Input: part model. Units: mm. Frame: model coordinates. Coordinates: 2 decimals unless noted, no trailing zeros. Loops run counter-clockwise (first coordinate to the right, second up) from the corner with the lowest first, then second, coordinate; pieces in that order, holes last. Notation, with made-up numbers: (77, 38.5) -> (125, 38.5) arc R24 cw to (125, 64.5) -> close; hole circle Ø7 at (43.25, 39.5). An arc over 180 degrees is marked (long way). Put each result on its own line as item: value. Start each with the question number.
1) Cut plane B-B (y = -111.5). Return the cut outline in (x, z), plus the area to 3 significant figures.
2) Cut plane A-A (z = 2.35). Return the cut outline in (x, y), plus the area to 3 significant figures.
3) Material intervals for L1, parallel to X at y = -190, z = 0.4; L2, parallel to Y at x = 71.5, z = 1.25; L3, parallel to X at y = -83, z = 2.1, sorted ascending.
4) Cut plane C-C (x = 137). Return the cut outline in (y, z), plus the area to 3 significant figures.
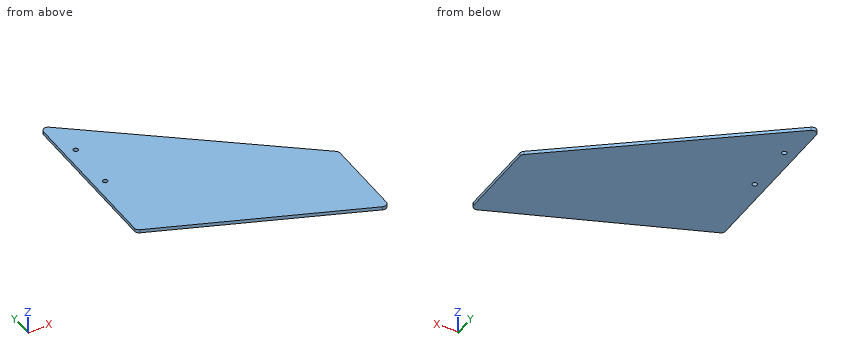
from build123d import *

# Parameters (mm, degrees)
EXTRUDE_1_DEPTH     = 3
FILLET_1_R          = 4
SKETCH_2_R          = 2.1
CUT_EXTRUDE_1_DEPTH = 3


with BuildPart() as part:
    # Эскиз1 → Бобышка-Вытянуть1 (new body)
    with BuildSketch(Plane.XY):
        Polygon((0, 0), (-3.068659699, -150), (178.455758645, -224), (180.065729767, -145.302558134), align=None)
    extrude(amount=EXTRUDE_1_DEPTH)

    # Скругление1
    fillet_1_edges = [part.edges().sort_by_distance(p)[0] for p in [
        (178.455758645, -224, 1.5),
        (-3.068659699, -150, 1.5),
        (0, 0, 1.5),
        (180.065729767, -145.302558134, 1.5),
    ]]
    fillet(fillet_1_edges, radius=FILLET_1_R)

    # Эскиз2 → Вырез-Вытянуть1 (cut)
    with BuildSketch(Plane.XY.offset(3)):
        with Locations((9.183783122, -40)):
            Circle(SKETCH_2_R)
        with Locations((8.259287105, -85.190544444)):
            Circle(SKETCH_2_R)
    extrude(amount=-CUT_EXTRUDE_1_DEPTH, mode=Mode.SUBTRACT)


solid = part.part
Results found:
1. outline: (-2.28, 0) -> (138.18, 0) -> (138.18, 3) -> (-2.28, 3) -> close
1. area: 421 mm2
2. outline: (-3.01, -147.25) arc R4 ccw to (-0.52, -151.04) -> (173.07, -221.8) arc R4 ccw to (178.57, -218.18) -> (180.03, -147.26) arc R4 ccw to (178.54, -144.07) -> (6.34, -5.12) arc R4 ccw to (-0.17, -8.15) -> close; hole circle Ø4.2 at (8.26, -85.19); hole circle Ø4.2 at (9.18, -40)
2. area: 20,900 mm2
3. L1: x = 95.05 to 179.15
3. L2: y = -180.4 to -57.7
3. L3: x = -1.7 to 102.86
4. outline: (-207.1, 0) -> (-110.55, 0) -> (-110.55, 3) -> (-207.1, 3) -> close
4. area: 290 mm2
